from build123d import *

# Parameters (mm, degrees)
SKETCH1_R     = 17.4
BODY_DEPTH    = 30
SKETCH2_R     = 8
SPIGOT_DEPTH  = 70
CHAMFERS_SIZE = 1
FILLET_2_R    = 1


with BuildPart() as part:
    # Sketch1 → Body (new body)
    with BuildSketch(Plane.XY):
        Circle(SKETCH1_R)
    extrude(amount=BODY_DEPTH)

    # Sketch2 → Spigot (add)
    with BuildSketch(Plane.XY.offset(30)):
        Circle(SKETCH2_R)
    extrude(amount=SPIGOT_DEPTH)

    # Chamfers
    chamfers_edges = [part.edges().sort_by_distance(p)[0] for p in [
        (-17.4, 0, 30),
        (-8, 0, 100),
    ]]
    chamfer(chamfers_edges, length=CHAMFERS_SIZE)

    # Fillet 2
    fillet_2_edges = [part.edges().sort_by_distance(p)[0] for p in [
        (-8, 0, 30),
    ]]
    fillet(fillet_2_edges, radius=FILLET_2_R)


solid = part.part
Here's how the part is built. I have some questions about the finished solid (model axes, mm). A direction names the side the tool comes from. Coordinates: 2 decimals unless noted, no trailing zeros. Write each loop counter-clockwise with the first axis right and the second up, starting at its lowest first coordinate (ties: lowest second). Pieces come first, ordered by that corner, then holes.
1) If we section it at C-C (z = 61): List the corners of the cut face in (x, y) for me.
Filled in:
outline: circle Ø16 at (0, 0)
2) I'm going to push flat-ended pins straight in: pin 1 (8 mm diameter, centred on x = -7, y = 5.5, fed in from +Z); pin 2 (8 mm diameter, centred on x = -4, y = -11.5, fed in from +Z); pin 3 (1 mm diameter, centred on y = -5.5, z = 35, fed in from -X) (3 decimals); pin 4 (1 mm diameter, centred on y = 6, z = 11, fed in from +X). Where does each tip first touch, or does it pass through?
Filled in:
pin 1: stops at z = 100
pin 2: stops at z = 30.43
pin 3: stops at x = -6.245
pin 4: stops at x = 16.51
3) If we section it at A-A (y = 0): List the corners of the cut face in (x, z) for me, plus the area to 3 significant figures.
Filled in:
outline: (-17.4, 0) - (17.4, 0) - (17.4, 29) - (16.4, 30) - (9, 30) arc R1 cw to (8, 31) - (8, 99) - (7, 100) - (-7, 100) - (-8, 99) - (-8, 31) arc R1 cw to (-9, 30) - (-16.4, 30) - (-17.4, 29) - close
area: 2,160 mm2
4) Which directions (+Z, -Z, +X, -X, +Y, -Y) give clear straight access to the entire face, cutting with the end or side of a thin tool? Please do faces 1 (the face through (7, -7, 30)), 2 (the face through (-3.772, -16.986, 14.297)).
Filled in:
face 1: +Z
face 2: +Z, -Z
5) If I drill on line 1 (Z direction, x = -4, y = -15); line 2 (X direction, y = 9.5, z = 14); line 3 (Y direction, x = 0, z = 61), over which ranges is the centre line in solid material (lowest first)?
Filled in:
line 1: z = 0 to 30
line 2: x = -14.58 to 14.58
line 3: y = -8 to 8
